Input: part model. Units: mm. Frame: model coordinates. Face numbers are marked on the shaded views. A direction names the side the tool comes from. Give positions to 0.01 mm unless a question says otherwise; leave off trailing zeros. Loops run counter-clockwise (first coordinate to the right, second up) from the corner with the lowest first, then second, coordinate; pieces in that order, holes last.
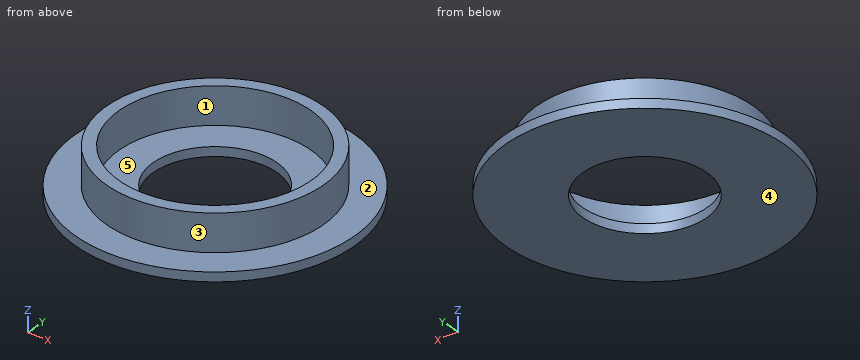
from build123d import *

# Parameters (mm, degrees)
SKETCH1_R           = 45
BOSS_EXTRUDE3_DEPTH = 3
SKETCH2_R           = 35
BOSS_EXTRUDE4_DEPTH = 12
SKETCH3_R           = 31
CUT_EXTRUDE2_DEPTH  = 12
SKETCH4_R           = 20
CUT_EXTRUDE3_DEPTH  = 8


with BuildPart() as part:
    # Sketch1 → Boss-Extrude3 (new body)
    with BuildSketch(Plane.XY):
        Circle(SKETCH1_R)
    extrude(amount=BOSS_EXTRUDE3_DEPTH)

    # Sketch2 → Boss-Extrude4 (add)
    with BuildSketch(Plane.XY.offset(3)):
        Circle(SKETCH2_R)
    extrude(amount=BOSS_EXTRUDE4_DEPTH)

    # Sketch3 → Cut-Extrude2 (cut)
    with BuildSketch(Plane.XY.offset(15)):
        Circle(SKETCH3_R)
    extrude(amount=-CUT_EXTRUDE2_DEPTH, mode=Mode.SUBTRACT)

    # Sketch4 → Cut-Extrude3 (cut)
    with BuildSketch(Plane.XY.offset(3)):
        Circle(SKETCH4_R)
    extrude(amount=-CUT_EXTRUDE3_DEPTH, mode=Mode.SUBTRACT)


solid = part.part
(1) Mould query, pull axis Y, two halves, no side actions, for the marked faces 1, 2 and 3. Classes: +Y half, -Y half, draft (parallel to the pull), parting line (faces both ways), or undercut.
Values follow:
face 1: undercut
face 2: draft
face 3: parting line
(2) Ray query, probe 1 along Y at (x, z) = (0, 0.95); probe 2 along Y at (x, z) = (0, 7.25); probe 3 along Z at (x, y) = (-11, -27.5). Return the intervals inside material, ascending.
Values follow:
probe 1: y = -45 to -20, 20 to 45
probe 2: y = -35 to -31, 31 to 35
probe 3: z = 0 to 3
(3) Reachability of the marked faces 4 and 5 from +Z, -Z, +X, -X, +Y, -Y: full face, straight path, thin tool, end or side. Return the list, or none.
Values follow:
face 4: -Z, +X, -X, +Y, -Y
face 5: +Z
(4) Pin query (flat end, axial travel): pin 1 Ø1.5 at (x, y) = (26.5, -28.5) entering from +Z; pin 2 Ø4 at (y, z) = (18.5, 9) entering from -X; pin 3 Ø6 at (y, z) = (3.5, 2) entering from -X. Return the tip coordinate at first contact, or that it passes through.
Values follow:
pin 1: stops at z = 3
pin 2: stops at x = -30.87
pin 3: stops at x = -45
(5) Cut plane A-A (x = 0). Return the cut outline in (y, z).
Values follow:
outline: (-45, 0) - (-20, 0) - (-20, 3) - (-31, 3) - (-31, 15) - (-35, 15) - (-35, 3) - (-45, 3) - close; (20, 0) - (45, 0) - (45, 3) - (35, 3) - (35, 15) - (31, 15) - (31, 3) - (20, 3) - close
(6) Cut plane C-C (z = 6). Return the cut outline in (x, y).
Values follow:
outline: circle Ø70 at (0, 0); hole circle Ø62 at (0, 0)
(7) Cut plane D-D (z = 1.25). Return the cut outline in (x, y).
Values follow:
outline: circle Ø90 at (0, 0); hole circle Ø40 at (0, 0)
